The listing builds one solid part. Answer for the finished solid, in the listing's coordinates (mm). Give positions to 0.01 mm unless a question says otherwise; leave off trailing zeros. Write each loop counter-clockwise with the first axis right and the second up, starting at its lowest first coordinate (ties: lowest second). Pieces come first, ordered by that corner, then holes. Notation, with made-up numbers: (-4, 65.25) -> (8, 65.25) arc R6 cw to (8, 76.25) -> close; hole circle Ø2 at (-30.75, -1). An arc over 180 degrees is marked (long way). Put each result on its own line as item: value. Start each with the question number.
1) Find the intervals of material crossed by line 1 along Y through (x, z) = (0, -0.1) (1 decimal); line 2 along Y through (x, z) = (11, -1.15) (1 decimal); line 3 along Y through (x, z) = (16, -0.05) (1 decimal), in increasing order. Write a range as from..to.
2) A cutting plane is placed at C-C (z = 0.55). Give the number of separate pieces and of enclosed holes in the cut face, then the cut area to 3 significant figures.
3) A cutting plane is placed at A-A (y = -75.5). Write down the section's boundary in (x, z), then the cut area to 3 significant figures.
4) A cutting plane is placed at B-B (x = 95). Write down the section's boundary in (y, z).
5) Flat-ended cylindrical pins translate along their axes: pin 1 Ø1.6 at (y, z) = (47, -0.5) entering from +X; pin 2 Ø1 at (y, z) = (96.5, 0) entering from -X; pin 3 Ø1 at (y, z) = (11, 1.5) entering from +X. Find the tip coordinate at first contact, or state that the pin passes through.
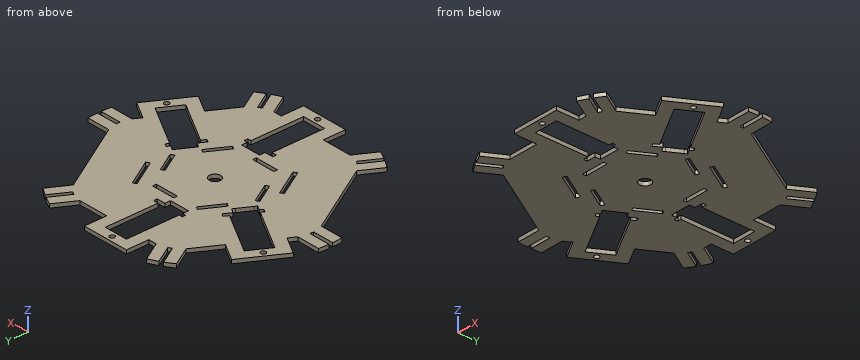
from build123d import *

# Parameters (mm, degrees)
SKETCH1_R                   = 110
SKETCH1_R_2                 = 4.7625
BOSS_EXTRUDE1_DEPTH         = 1.5875
SKETCH2_R                   = 2.15375
CUT_EXTRUDE3_DEPTH          = 4.175
CIRPATTERN1_COUNT           = 2
CIRPATTERN2_COUNT           = 2
CIRPATTERN2_ANGLE           = 60
CIRPATTERN2_COPY_1_SKETCH_R = 2.15375
CIRPATTERN2_COPY_1_DEPTH    = 4.175
CUT_EXTRUDE5_DEPTH          = 4.175
CUT_EXTRUDE8_DEPTH          = 5
SKETCH11_W                  = 27.2625
SKETCH11_H                  = 3.175
SKETCH11_W_2                = 20
CUT_EXTRUDE24_DEPTH         = 5


with BuildPart() as part:
    # Sketch1 → Boss-Extrude1 (new body, symmetric)
    with BuildSketch(Plane.XY):
        Circle(SKETCH1_R)
        Circle(SKETCH1_R_2, mode=Mode.SUBTRACT)
        Polygon((-4.7625, 40), (-2.2625, 40), (-2.2625, 48), (0.7375, 48), (0.7375, 93), (-19.2625, 93), (-19.2625, 40), (-16.7625, 40), align=None, mode=Mode.SUBTRACT)
        Polygon((4.7625, -40), (2.2625, -40), (2.2625, -48), (-0.7375, -48), (-0.7375, -93), (19.2625, -93), (19.2625, -40), (16.7625, -40), align=None, mode=Mode.SUBTRACT)
        Polygon((37.022266151, -15.875554014), (35.772266151, -18.040617524), (42.700469382, -22.040617524), (41.200469382, -24.638693735), (80.171612552, -47.138693735), (90.171612552, -29.81818566), (44.272266151, -3.31818566), (43.022266151, -5.483249169), align=None, mode=Mode.SUBTRACT)
        Polygon((-37.022266151, 15.875554014), (-35.772266151, 18.040617524), (-42.700469382, 22.040617524), (-41.200469382, 24.638693735), (-80.171612552, 47.138693735), (-90.171612552, 29.81818566), (-44.272266151, 3.31818566), (-43.022266151, 5.483249169), align=None, mode=Mode.SUBTRACT)
    extrude(amount=BOSS_EXTRUDE1_DEPTH, both=True)

    # Sketch2 → Cut-Extrude3 (cut, through all)
    with BuildSketch(Plane.XY.offset(1.5875)):
        with Locations((10.7625, -97.43875)):
            Circle(SKETCH2_R)
        with BuildLine():
            Line((-10.7375, -82.808492409), (-10.7375, -101.88))
            Line((-10.7375, -101.88), (9.2625, -101.88))
            Line((9.2625, -101.88), (29.2625, -101.88))
            Line((29.2625, -101.88), (29.2625, -82.808492409))
            Line((29.2625, -82.808492409), (36.2625, -82.808492409))
            Line((36.2625, -82.808492409), (46.112001713, -99.868329805))
            ThreePointArc((46.112001713, -99.868329805), (0, -110), (-46.112001713, -99.868329805))
            Line((-46.112001713, -99.868329805), (-36.2625, -82.808492409))
            Line((-36.2625, -82.808492409), (-10.7375, -82.808492409))
        make_face()
    cut_extrude3 = extrude(amount=-CUT_EXTRUDE3_DEPTH, mode=Mode.SUBTRACT)

    # CirPattern1: Cut-Extrude3 ×2 about axis
    cirpattern1_axis = Axis((0, 0, 0), (0, 0, 1))
    for i in range(1, CIRPATTERN1_COUNT):
        add(cut_extrude3.rotate(cirpattern1_axis, i * 360 / CIRPATTERN1_COUNT), mode=Mode.SUBTRACT)

    # CirPattern2: Cut-Extrude3 ×2 about axis
    cirpattern2_axis = Axis((0, 0, 0), (0, 0, 1))
    for i in range(1, CIRPATTERN2_COUNT):
        add(cut_extrude3.rotate(cirpattern2_axis, i * CIRPATTERN2_ANGLE / (CIRPATTERN2_COUNT - 1)), mode=Mode.SUBTRACT)

    # CirPattern2 copy 1 sketch → CirPattern2 copy 1 (cut, through all)
    with BuildSketch(Plane(origin=(0, 0, 1.5875), x_dir=(-0.5, -0.866025404, 0), z_dir=(0, 0, 1))):
        with Locations((10.7625, -97.43875)):
            Circle(CIRPATTERN2_COPY_1_SKETCH_R)
        with BuildLine():
            Line((-10.7375, -82.808492409), (-10.7375, -101.88))
            Line((-10.7375, -101.88), (9.2625, -101.88))
            Line((9.2625, -101.88), (29.2625, -101.88))
            Line((29.2625, -101.88), (29.2625, -82.808492409))
            Line((29.2625, -82.808492409), (36.2625, -82.808492409))
            Line((36.2625, -82.808492409), (46.112001713, -99.868329805))
            ThreePointArc((46.112001713, -99.868329805), (0, -110), (-46.112001713, -99.868329805))
            Line((-46.112001713, -99.868329805), (-36.2625, -82.808492409))
            Line((-36.2625, -82.808492409), (-10.7375, -82.808492409))
        make_face()
    extrude(amount=-CIRPATTERN2_COPY_1_DEPTH, mode=Mode.SUBTRACT)

    # Sketch5 → Cut-Extrude5 (cut, through all)
    with BuildSketch(Plane.XY.offset(1.5875)):
        with BuildLine():
            Line((89.845508076, 10), (53.583008076, 72.808492409))
            Line((53.583008076, 72.808492409), (63.432509788, 89.868329805))
            ThreePointArc((63.432509788, 89.868329805), (95.262794416, 55), (109.544511501, 10))
            Line((109.544511501, 10), (89.845508076, 10))
        make_face()
        with BuildLine():
            Line((-89.845508076, -10), (-53.583008076, -72.808492409))
            Line((-53.583008076, -72.808492409), (-63.432509788, -89.868329805))
            ThreePointArc((-63.432509788, -89.868329805), (-95.262794416, -55), (-109.544511501, -10))
            Line((-109.544511501, -10), (-89.845508076, -10))
        make_face()
    extrude(amount=-CUT_EXTRUDE5_DEPTH, mode=Mode.SUBTRACT)

    # Sketch10 → Cut-Extrude8 (cut, symmetric)
    with BuildSketch(Plane.XY.offset(1.5875)):
        Polygon((-65.369087402, -110.047580625), (-56.369087402, -94.459123357), (-47.369087402, -78.870666089), (-44.619456745, -80.458166089), (-53.619456745, -96.046623357), (-62.619456745, -111.635080625), align=None)
        Polygon((-127.988544148, 1.5875), (-109.988544148, 1.5875), (-91.988544148, 1.5875), (-91.988544148, -1.5875), (-109.988544148, -1.5875), (-127.988544148, -1.5875), align=None)
        Polygon((-62.619456745, 111.635080625), (-53.619456745, 96.046623357), (-44.619456745, 80.458166089), (-47.369087402, 78.870666089), (-56.369087402, 94.459123357), (-65.369087402, 110.047580625), align=None)
        Polygon((65.369087402, 110.047580625), (56.369087402, 94.459123357), (47.369087402, 78.870666089), (44.619456745, 80.458166089), (53.619456745, 96.046623357), (62.619456745, 111.635080625), align=None)
        Polygon((127.988544148, -1.5875), (109.988544148, -1.5875), (91.988544148, -1.5875), (91.988544148, 1.5875), (109.988544148, 1.5875), (127.988544148, 1.5875), align=None)
        Polygon((62.619456745, -111.635080625), (53.619456745, -96.046623357), (44.619456745, -80.458166089), (47.369087402, -78.870666089), (56.369087402, -94.459123357), (65.369087402, -110.047580625), align=None)
    extrude(amount=CUT_EXTRUDE8_DEPTH, both=True, mode=Mode.SUBTRACT)

    # Sketch11 → Cut-Extrude24 (cut, symmetric)
    with BuildSketch(Plane.XY.offset(1.5875)):
        with Locations((8.63125, -46.4125)):
            Rectangle(SKETCH11_W, SKETCH11_H)
        Polygon((-44.069219382, -19.669872981), (-30.437969382, -43.279890552), (-27.688338725, -41.692390552), (-41.319588725, -18.082372981), align=None)
        with Locations((-9.06699264, -34.6125)):
            Rectangle(SKETCH11_W_2, SKETCH11_H)
        Polygon((-38.13398528, 0), (-40.883615937, -1.5875), (-30.883615937, -18.908008076), (-28.13398528, -17.320508076), align=None)
        Polygon((-39.069219382, 28.330127019), (-52.700469382, 4.720109448), (-49.950838725, 3.132609448), (-36.319588725, 26.742627019), align=None)
        Polygon((-19.06699264, 33.025), (-21.816623297, 34.6125), (-31.816623297, 17.291991924), (-29.06699264, 15.704491924), align=None)
        with Locations((-8.63125, 46.4125)):
            Rectangle(SKETCH11_W, SKETCH11_H)
        with Locations((9.06699264, 34.6125)):
            Rectangle(SKETCH11_W_2, SKETCH11_H)
        Polygon((44.069219382, 19.669872981), (30.437969382, 43.279890552), (27.688338725, 41.692390552), (41.319588725, 18.082372981), align=None)
        Polygon((38.13398528, 0), (40.883615937, 1.5875), (30.883615937, 18.908008076), (28.13398528, 17.320508076), align=None)
        Polygon((39.069219382, -28.330127019), (52.700469382, -4.720109448), (49.950838725, -3.132609448), (36.319588725, -26.742627019), align=None)
        Polygon((19.06699264, -33.025), (21.816623297, -34.6125), (31.816623297, -17.291991924), (29.06699264, -15.704491924), align=None)
    extrude(amount=CUT_EXTRUDE24_DEPTH, both=True, mode=Mode.SUBTRACT)


solid = part.part
Reply:
1. line 1: y = -101.9..-93, -44.8..-36.2, -33..-4.8, 4.8..33, 36.2..44.8, 93..101.9
1. line 2: y = -101.9..-99.6, -95.3..-93, -40..33, 36.2..82.8
1. line 3: y = -101.9..-93, -40..33, 36.2..82.8
2. separate pieces: 1
2. enclosed holes: 17
2. area: 23,600 mm2
3. outline: (-55.14, -1.59) -> (-0.74, -1.59) -> (-0.74, 1.59) -> (-55.14, 1.59) -> close; (19.26, -1.59) -> (55.14, -1.59) -> (55.14, 1.59) -> (19.26, 1.59) -> close
3. area: 287 mm2
4. outline: (-39.22, -1.59) -> (-21.06, -1.59) -> (-21.06, 1.59) -> (-39.22, 1.59) -> close; (-10, -1.59) -> (-1.59, -1.59) -> (-1.59, 1.59) -> (-10, 1.59) -> close; (1.59, -1.59) -> (10, -1.59) -> (10, 1.59) -> (1.59, 1.59) -> close
5. pin 1: stops at x = 68.95
5. pin 2: stops at x = -53.62
5. pin 3: stops at x = 89.56
